The listing builds one solid part. Answer for the finished solid, in the listing's coordinates (mm). Face numbers are marked on the shaded views. A direction names the side the tool comes from. Coordinates: 2 decimals unless noted, no trailing zeros. Order: outer loops, then holes, each group sorted by start corner. A loop starts at its lowest first (then second) coordinate and runs counter-clockwise, first axis right, second up. Notation, with made-up numbers: (-7, 61) -> (0, 61) arc R21 ccw to (0, 82) -> close; hole circle Ø7 at (81, 27.5). An arc over 180 degrees is marked (long way). Return JSON: item names as keys, results as strings.
from build123d import *

# Parameters (mm, degrees)
F0_R            = 61.5853666469
F1_DEPTH        = 25
F2_R            = 17.4311755098
F3_DEPTH        = 25
F5_DEPTH        = 25
F5_COPIES_COUNT = 12


# Not quite as in the source:
# - a pattern or mirror of a feature is missing from the dataset's text; its kind, count and spacing are read off the source's solid


with BuildPart() as f1:
    # F0 (on Top) → F1 (new body)
    with BuildSketch(Plane.XY):
        Circle(F0_R)
    extrude(amount=F1_DEPTH)

    # F2 (on face) → F3 (cut)
    with BuildSketch(Plane.XY.offset(25)):
        Circle(F2_R)
    extrude(amount=-F3_DEPTH, mode=Mode.SUBTRACT)

    # F4 (on Top) → F5 (join)
    with BuildSketch(Plane.XY):
        with BuildLine():
            Line((0, 85), (-12.9957382045, 60.1985728532))
            ThreePointArc((-12.9957382045, 60.1985728532), (0, 61.5853666469), (12.9957382045, 60.1985728532))
            Line((12.9957382045, 60.1985728532), (0, 85))
        make_face()
    f5 = extrude(amount=F5_DEPTH)

    # F5_copies: F5 ×12 about axis
    f5_copies_axis = Axis((0, 0, 0), (0, 0, 1))
    for i in range(1, F5_COPIES_COUNT):
        add(f5.rotate(f5_copies_axis, i * 360 / F5_COPIES_COUNT))


solid = f1.part
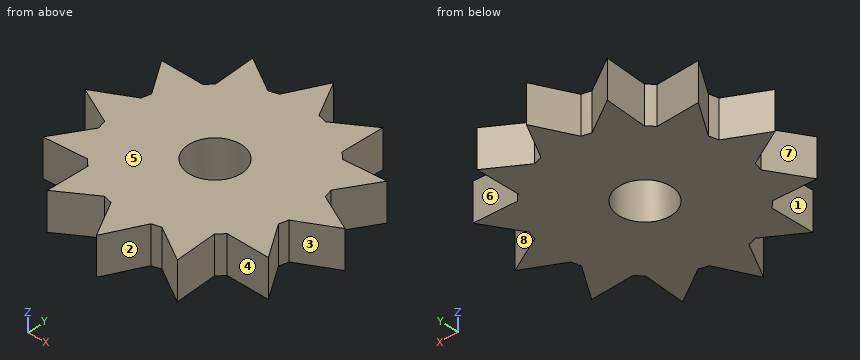
1. Determine the mould class of the marked faces 1, 2 and 3 for opening direction X: pulls with the +X half, pulls with the -X half, needs draft (parallel to the pull), parting line crosses it, or undercut.
Answer block:
{"face 1": "pulls with the -X half", "face 2": "undercut", "face 3": "pulls with the +X half"}
2. The part is cut by section A-A on x = 24.5. Give the vertices of the cut face in (y, z), and give its area (3 significant figures).
Answer block:
{"outline": "(-62.21, 0) -> (62.21, 0) -> (62.21, 25) -> (-62.21, 25) -> close", "area": "3,110 mm2"}
3. Consider line 1 (Y direction, x = -63, z = 18.75); line 2 (Y direction, x = 0, z = 12); line 3 (Y direction, x = 69, z = 9.5). Determine where each line is inside the solid, lowest interval first. Write a range as from..to.
Answer block:
{"line 1": "y = -42.07..-25.74, -11.53..11.53, 25.74..42.07", "line 2": "y = -85..-17.43, 17.43..85", "line 3": "y = -42.31..-35.22, -8.38..8.38, 35.22..42.31"}
4. Each of these flat-tipped pins is pushed along its axis until it touches: pin 1 Ø1.5 at (y, z) = (22, 12.5) entering from +X; pin 2 Ø4 at (y, z) = (-10, 16) entering from +X; pin 3 Ø1 at (x, z) = (63.5, 22) entering from +Y; pin 4 Ø5 at (x, y) = (-22.5, -36) entering from -Z. Where does it stop, or does it pass through?
Answer block:
{"pin 1": "stops at x = 61.1", "pin 2": "stops at x = 69.73", "pin 3": "stops at y = 42.11", "pin 4": "stops at z = 0"}
5. For the marked faces 4, 5, 6, 7 and 8, determine the directions among +Z, -Z, +X, -X, +Y, -Y from which every point of the face is accessible in a straight line to the end or side of a thin tool.
Answer block:
{"face 4": "+Z, -Z, -Y", "face 5": "+Z, +X, -X, +Y, -Y", "face 6": "+Z, -Z, +Y", "face 7": "+Z, -Z, -X", "face 8": "+Z, -Z, +X"}
